Source: three-view drawing plus pictorial views. Frame: mm from the lowest corner of the part. A direction names the side the tool comes from. Coordinates: 2 decimals unless noted, no trailing zeros. Write each loop counter-clockwise with the first axis right and the second up, starting at its lowest first coordinate (ties: lowest second). Pieces come first, ordered by that corner, then holes. Notation, with made-up numbers: (43.5, 17.25) - (98.5, 17.25) arc R33 cw to (98.5, 55.25) - close; hole circle Ø4 at (17.25, 21.25). An arc over 180 degrees is marked (long way). Put each result on its own line as item: value.
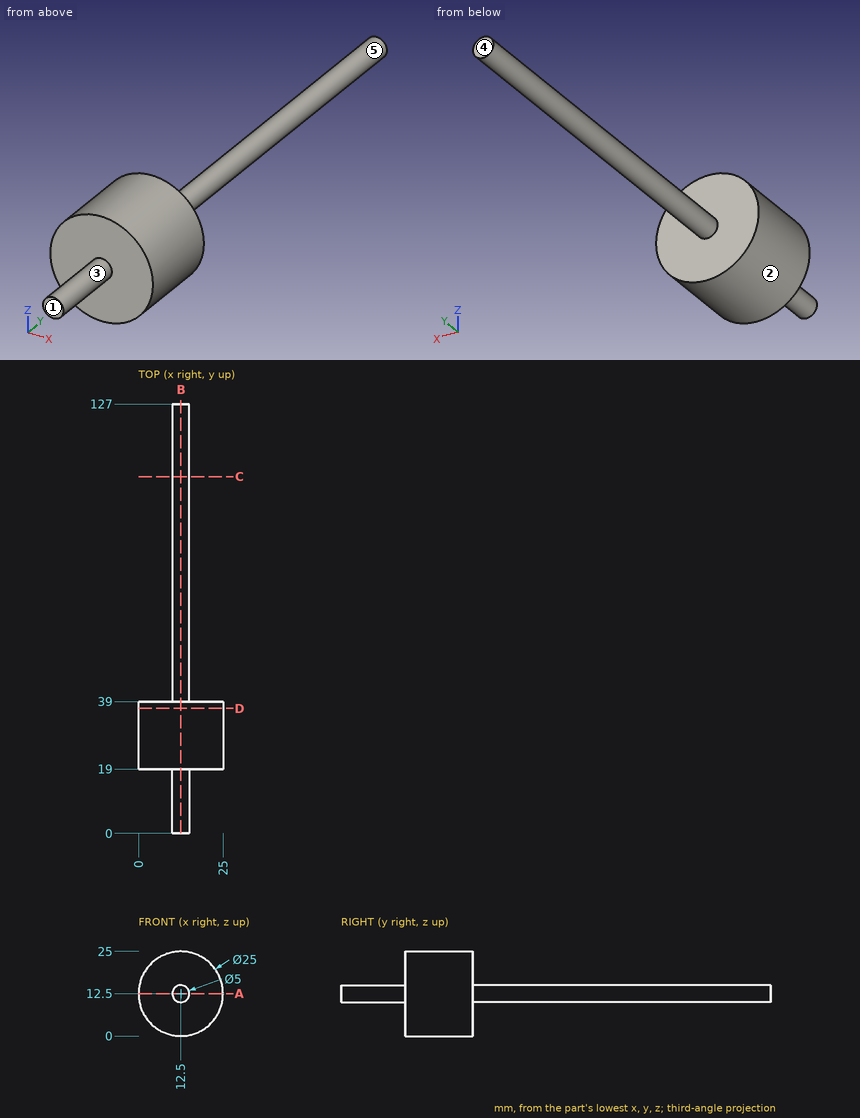
1. Section query D-D (y = 37). Return loops of the section in (x, z).
Answer below:
outline: circle Ø25 at (12.5, 12.5)
2. Ray query, probe 1 along Y at (x, z) = (11.5, 16.75); probe 2 along Z at (x, y) = (12.5, 42.5); probe 3 along X at (y, z) = (36, 1.5). Return the intervals inside material, ascending. Write a range as from..to.
Answer below:
probe 1: y = 19..39
probe 2: z = 10..15
probe 3: x = 6.56..18.44
3. Section query A-A (z = 12.5). Return loops of the section in (x, y), then the cut area to 4 significant figures.
Answer below:
outline: (0, 19) - (10, 19) - (10, 0) - (15, 0) - (15, 19) - (25, 19) - (25, 39) - (15, 39) - (15, 127) - (10, 127) - (10, 39) - (0, 39) - close
area: 1,035 mm²
4. Section query C-C (y = 105.5). Return loops of the section in (x, z), then the cut area to 3 significant figures.
Answer below:
outline: circle Ø5 at (12.5, 12.5)
area: 19.6 mm²
5. Section query B-B (x = 12.5). Return loops of the section in (y, z).
Answer below:
outline: (0, 10) - (19, 10) - (19, 0) - (39, 0) - (39, 10) - (127, 10) - (127, 15) - (39, 15) - (39, 25) - (19, 25) - (19, 15) - (0, 15) - close
6. Mould query, pull axis X, two halves, no side actions, for the marked faces 1 and 2. Classes: +X half, -X half, draft (parallel to the pull), parting line (faces both ways), or undercut.
Answer below:
face 1: draft
face 2: parting line
7. Set-up query: the marked faces 3, 4 and 5. Return all of +Z, -Z, +X, -X, +Y, -Y with unobstructed straight access to the full face (end or side cutting, diameter ignored); none if empty.
Answer below:
face 3: -Y
face 4: +Z, -Z, +X, -X, +Y
face 5: +Y
8. Pin query (flat end, axial travel): pin 1 Ø3 at (x, z) = (13, 19) entering from +Y; pin 2 Ø8 at (x, z) = (19.5, 3) entering from -Y; pin 3 Ø5 at (x, z) = (9.5, 14.5) entering from -Y; pin 4 Ø6 at (x, y) = (11.5, 73.5) entering from -Z. Return the tip coordinate at first contact, or that it passes through.
Answer below:
pin 1: stops at y = 39
pin 2: stops at y = 19
pin 3: stops at y = 0
pin 4: stops at z = 10
